Geometry check sheet. Reference: the model listing, model coordinates, mm. Round coordinates to 2 decimals unless told otherwise and drop trailing zeros. Write each loop counter-clockwise with the first axis right and the second up, starting at its lowest first coordinate (ties: lowest second). Pieces come first, ordered by that corner, then holes. Notation, with made-up numbers: M 17.5,4 L 76.5,4 A15 ccw 76.5,25 Z; hole C -35.5,18.25 d7. An arc over 180 degrees is marked long. One line per item, written item: value. Start each with the question number.
1. Scan lines: probe 1 along Y at (x, z) = (0, 2.1); probe 2 along Y at (x, z) = (-24.25, 1.5); probe 3 along Y at (x, z) = (-35, 1.7). Record each from-to range of solid material in increasing order. Write a range as [from, to].
2. Section check A-A (x = -35). Record the boundary of the cut face in (y, z).
3. Section check B-B (x = 0). Count the separate pieces of the cut face and the enclosed holes in it, and give its area (3 significant figures).
from build123d import *

# Parameters (mm, degrees)
F0_W     = 97
F0_H     = 50
F0_R     = 2.5
F0_R_2   = 3
F0_R_3   = 10
F1_DEPTH = 4
F2_R     = 2
F3_SIZE  = 0.49999


# Not quite as in the source:
# - a fillet or chamfer is up to 0.001 mm smaller than in the source, because OpenCascade refuses the exact size


with BuildPart() as f1:
    # F0 (on Top) → F1 (new body)
    with BuildSketch(Plane.XY):
        Rectangle(F0_W, F0_H)
        with Locations((-44.5, -21)):
            Circle(F0_R, mode=Mode.SUBTRACT)
        with Locations((-42.7, -13)):
            Circle(F0_R_2, mode=Mode.SUBTRACT)
        with Locations((-24.25, -21)):
            Circle(F0_R, mode=Mode.SUBTRACT)
        with Locations((-12.3, -13)):
            Circle(F0_R_2, mode=Mode.SUBTRACT)
        with Locations((0, -21)):
            Circle(F0_R_2, mode=Mode.SUBTRACT)
        with Locations((12.3, -13)):
            Circle(F0_R_2, mode=Mode.SUBTRACT)
        with Locations((24.25, -21)):
            Circle(F0_R, mode=Mode.SUBTRACT)
        with Locations((44.5, -21)):
            Circle(F0_R, mode=Mode.SUBTRACT)
        with Locations((42.7, -13)):
            Circle(F0_R_2, mode=Mode.SUBTRACT)
        with Locations((-35, 0)):
            Circle(F0_R_2, mode=Mode.SUBTRACT)
        with Locations((-24.25, 0)):
            Circle(F0_R_2, mode=Mode.SUBTRACT)
        with Locations((-15, 0)):
            Circle(F0_R_2, mode=Mode.SUBTRACT)
        with Locations((-42.7, 13)):
            Circle(F0_R_2, mode=Mode.SUBTRACT)
        with Locations((-44.5, 21)):
            Circle(F0_R, mode=Mode.SUBTRACT)
        with Locations((-12.3, 13)):
            Circle(F0_R_2, mode=Mode.SUBTRACT)
        with Locations((-24.25, 21)):
            Circle(F0_R, mode=Mode.SUBTRACT)
        Circle(F0_R_3, mode=Mode.SUBTRACT)
        with Locations((15, 0)):
            Circle(F0_R_2, mode=Mode.SUBTRACT)
        with Locations((24.25, 0)):
            Circle(F0_R_2, mode=Mode.SUBTRACT)
        with Locations((35, 0)):
            Circle(F0_R_2, mode=Mode.SUBTRACT)
        with Locations((12.3, 13)):
            Circle(F0_R_2, mode=Mode.SUBTRACT)
        with Locations((0, 21)):
            Circle(F0_R, mode=Mode.SUBTRACT)
        with Locations((42.7, 13)):
            Circle(F0_R_2, mode=Mode.SUBTRACT)
        with Locations((24.25, 21)):
            Circle(F0_R, mode=Mode.SUBTRACT)
        with Locations((44.5, 21)):
            Circle(F0_R, mode=Mode.SUBTRACT)
    extrude(amount=F1_DEPTH)

    # F2
    f2_edges = [f1.edges().sort_by_distance(p)[0] for p in [
        (-48.5, 25, 2),
        (-48.5, -25, 2),
        (48.5, -25, 2),
        (48.5, 25, 2),
    ]]
    fillet(f2_edges, radius=F2_R)

    # F3 (size 0.5 in the source; OpenCascade refuses exactly that, so slightly less here)
    f3_edges = [f1.edges().sort_by_distance(p)[0] for p in [
        (0, -25, 4),
        (-47.914214, -24.414214, 4),
        (47.914214, -24.414214, 4),
        (-48.5, 0, 4),
        (48.5, 0, 4),
        (-47.914214, 24.414214, 4),
        (47.914214, 24.414214, 4),
        (0, 25, 4),
        (-47, -21, 4),
        (-45.7, -13, 4),
        (-26.75, -21, 4),
        (-15.3, -13, 4),
        (-3, -21, 4),
        (9.3, -13, 4),
        (21.75, -21, 4),
        (42, -21, 4),
        (39.7, -13, 4),
        (-38, 0, 4),
        (-27.25, 0, 4),
        (-18, 0, 4),
        (-45.7, 13, 4),
        (-47, 21, 4),
        (-15.3, 13, 4),
        (-26.75, 21, 4),
        (-10, 0, 4),
        (12, 0, 4),
        (21.25, 0, 4),
        (32, 0, 4),
        (9.3, 13, 4),
        (-2.5, 21, 4),
        (39.7, 13, 4),
        (21.75, 21, 4),
        (42, 21, 4),
        (0, -25, 0),
        (-47.914214, -24.414214, 0),
        (47.914214, -24.414214, 0),
        (-48.5, 0, 0),
        (48.5, 0, 0),
        (-47.914214, 24.414214, 0),
        (47.914214, 24.414214, 0),
        (0, 25, 0),
        (-47, -21, 0),
        (-45.7, -13, 0),
        (-26.75, -21, 0),
        (-15.3, -13, 0),
        (-3, -21, 0),
        (9.3, -13, 0),
        (21.75, -21, 0),
        (42, -21, 0),
        (39.7, -13, 0),
        (-38, 0, 0),
        (-27.25, 0, 0),
        (-18, 0, 0),
        (-45.7, 13, 0),
        (-47, 21, 0),
        (-15.3, 13, 0),
        (-26.75, 21, 0),
        (-10, 0, 0),
        (12, 0, 0),
        (21.25, 0, 0),
        (32, 0, 0),
        (9.3, 13, 0),
        (-2.5, 21, 0),
        (39.7, 13, 0),
        (21.75, 21, 0),
        (42, 21, 0),
    ]]
    chamfer(f3_edges, length=F3_SIZE)


solid = f1.part
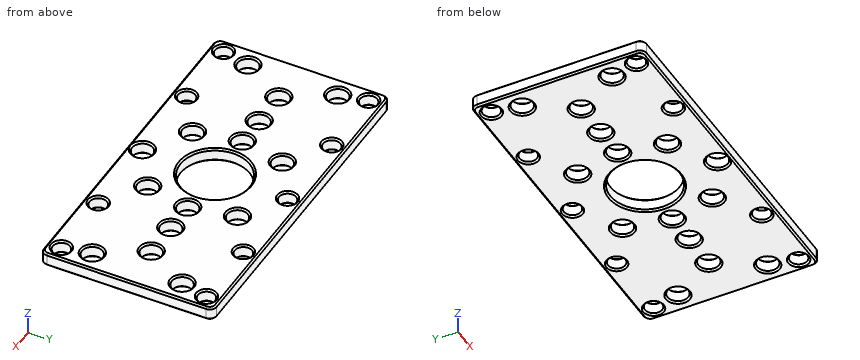
Result sheet:
1. probe 1: y = [-25, -24], [-18, -10], [10, 18.5], [23.5, 25]
1. probe 2: y = [-25, -23.5], [-18.5, -3], [3, 18.5], [23.5, 25]
1. probe 3: y = [-25, -3], [3, 25]
2. outline: M -25,0.5 L -24.5,0 L -3.5,0 L -3,0.5 L -3,3.5 L -3.5,4 L -24.5,4 L -25,3.5 Z; M 3,0.5 L 3.5,0 L 24.5,0 L 25,0.5 L 25,3.5 L 24.5,4 L 3.5,4 L 3,3.5 Z
3. separate pieces: 4
3. enclosed holes: 0
3. area: 74.0 mm2
